from build123d import *

# Parameters (mm, degrees)
F1_DEPTH  = 8.6
F2_R      = 12
F3_R      = 8
F4_R      = 15
F5_R      = 5
F6_R      = 5
F7_R      = 2
F8_R      = 2
F9_DEPTH  = 25
F11_START = -6
F10_R     = 3.6
F11_DEPTH = 19


with BuildPart() as f1:
    # F0 (on Front) → F1 (new body)
    with BuildSketch(Plane.XZ):
        Polygon((0, 120), (0, 0), (10, 0), (17.5520956899, 108), (55, 108), (55, 133), (49, 133), (44.2683869545, 120), align=None)
    extrude(amount=F1_DEPTH)

    # F2
    f2_edges = [f1.edges().sort_by_distance(p)[0] for p in [
        (17.552096, -4.3, 108),
    ]]
    fillet(f2_edges, radius=F2_R)

    # F3
    f3_edges = [f1.edges().sort_by_distance(p)[0] for p in [
        (10, -4.3, 0),
    ]]
    fillet(f3_edges, radius=F3_R)

    # F4
    f4_edges = [f1.edges().sort_by_distance(p)[0] for p in [
        (0, -4.3, 120),
    ]]
    fillet(f4_edges, radius=F4_R)

    # F5
    f5_edges = [f1.edges().sort_by_distance(p)[0] for p in [
        (55, -4.3, 108),
    ]]
    fillet(f5_edges, radius=F5_R)

    # F6
    f6_edges = [f1.edges().sort_by_distance(p)[0] for p in [
        (44.268387, -4.3, 120),
    ]]
    fillet(f6_edges, radius=F6_R)

    # F7
    f7_edges = [f1.edges().sort_by_distance(p)[0] for p in [
        (49, -4.3, 133),
        (55, -4.3, 133),
    ]]
    fillet(f7_edges, radius=F7_R)

    # F8 (on face) → F9 (cut)
    with BuildSketch(Plane(origin=(0, 0, 0), x_dir=(0, -1, 0), z_dir=(-1, 0, 0))):
        with Locations((4.3, 80)):
            Circle(F8_R)
    extrude(amount=-F9_DEPTH, mode=Mode.SUBTRACT)

    # F10 (on face) → F11 (cut)
    with BuildSketch(Plane(origin=(0, 0, 0), x_dir=(0, -1, 0), z_dir=(-1, 0, 0)).offset(F11_START)):
        with Locations((4.3, 80)):
            Circle(F10_R)
    extrude(amount=-F11_DEPTH, mode=Mode.SUBTRACT)


solid = f1.part
Model file for the job. Use its own axes, mm. A direction names the side the tool comes from. Give positions to 0.01 mm unless a question says otherwise; leave off trailing zeros. Order: outer loops, then holes, each group sorted by start corner. A loop starts at its lowest first (then second) coordinate and runs counter-clockwise, first axis right, second up. Notation, with made-up numbers: (-24, 85.5) - (-13, 85.5) arc R22 ccw to (-13, 116.5) - close; hole circle Ø8 at (-15.75, 22). An arc over 180 degrees is marked (long way). Return JSON: item names as keys, results as strings.
1) Cut at A-A, the plane y = -4.3. Give the cut face in (x, z).
Geometry says:
{"outline": "(0, 0) - (2.54, 0) arc R8 ccw to (10.52, 7.44) - (15.34, 76.4) - (6, 76.4) - (6, 78) - (0, 78) - close; (0, 82) - (6, 82) - (6, 83.6) - (15.85, 83.6) - (16.77, 96.84) arc R12 cw to (28.74, 108) - (50, 108) arc R5 ccw to (55, 113) - (55, 131) arc R2 ccw to (53, 133) - (50.4, 133) arc R2 ccw to (48.52, 131.68) - (45.47, 123.29) arc R5 cw to (40.77, 120) - (15, 120) arc R15 ccw to (0, 105) - close"}
2) Cut at D-D, the plane z = 41. Give the cut face in (x, y), plus the area to 3 significant figures.
Geometry says:
{"outline": "(0, -8.6) - (12.87, -8.6) - (12.87, 0) - (0, 0) - close", "area": "111 mm²"}
3) Flat gauge pins, fed straight in: P1, Ø1.5, axis at y = -4, z = 73, coming from the +X side; P2, Ø3, axis at x = 32, y = -1, coming from the -Z side; P3, Ø3, axis at x = 26.5, y = -6.5, coming from the +Z side; P4, Ø3, axis at y = -4.3, z = 80, coming from the -X side. Where does each tip first touch, or does it go through?
Geometry says:
{"P1": "x = 15.16", "P2": "z = 108", "P3": "z = 120", "P4": "through"}
4) Pull direction Y, two halves, no side cores. Call faces 4 (the flat face through (39, -4, 108)), 5 (the cylindrical face through (2.958, -4.04, 81.983)), 6 (the flat face through (15, 0, 82)): pulls with the +Y half, pulls with the -Y half, needs draft (parallel to the pull), parting line crosses it, or undercut.
Geometry says:
{"face 4": "needs draft", "face 5": "undercut", "face 6": "pulls with the +Y half"}
5) Cut at C-C, the plane x = 35. Give the cut face in (y, z).
Geometry says:
{"outline": "(-8.6, 108) - (0, 108) - (0, 120) - (-8.6, 120) - close"}
6) Cut at B-B, the plane z = 80. Give the cut face in (x, y), plus the area to 3 significant figures.
Geometry says:
{"outline": "(0, -8.6) - (15.59, -8.6) - (15.59, -7.9) - (6, -7.9) - (6, -6.3) - (0, -6.3) - close; (0, -2.3) - (6, -2.3) - (6, -0.7) - (15.59, -0.7) - (15.59, 0) - (0, 0) - close", "area": "41.0 mm²"}
7) 3-axis set-ups, long thin cutter, end or side, ignore diameter. For faces 1 (the flat face through (28, -4, 120)), 2 (the flat face through (55, -4, 122)), 3 (the flat face through (6, -6, 78)): which of +Z, -Z, +X, -X, +Y, -Y reach the whole face in a straight line?
Geometry says:
{"face 1": "+Z, -X, +Y, -Y", "face 2": "+Z, -Z, +X, +Y, -Y", "face 3": "+X"}
8) Probe line 1 (Y direction, x = 10, z = 80); line 2 (Z direction, x = 29, y = -3); line 3 (Z direction, x = 3.1, y = -4.3). List the from-to ranges inside material, lowest first. Write a range as from..to.
Geometry says:
{"line 1": "-8.6..-7.9, -0.7..0", "line 2": "108..120", "line 3": "0.02..78, 82..114.13"}
